Autodesk Fusion 360 part; units mm, degrees
sketch "Schizzo1" plane through (0, 0, 0) normal (0, 0, 1) x (1, 0, 0)
  line L0 (0, 0) -> (200, 0)
  line L1 (200, 0) -> (200, 200)
  line L2 (200, 200) -> (0, 200)
  line L3 (0, 200) -> (0, 0)
  line L4 (0, 100) -> (200, 100) construction
  line L5 (200, 100) -> (220, 100) construction
  line L6 (0, 100) -> (-20, 100) construction
  line L7 (220, 100) -> (220, 190.15)
  line L8 (220, 190.15) -> (200, 190.15)
  line L9 (220, 100) -> (220, 9.85)
  line L10 (220, 9.85) -> (200, 9.85)
  line L11 (-20, 100) -> (-20, 190.15)
  line L12 (-20, 190.15) -> (0, 190.15)
  line L13 (-20, 100) -> (-20, 9.85)
  line L14 (-20, 9.85) -> (0, 9.85)
  line L15 (0, 190.15) -> (200, 190.15) construction
  line L16 (200, 9.85) -> (0, 9.85) construction
  line L17 (0, 49.85) -> (200, 49.85) construction
  line L18 (122, 71.85) -> (78, 71.85)
  line L19 (78, 71.85) -> (78, 27.85)
  line L20 (78, 27.85) -> (122, 27.85)
  line L21 (122, 27.85) -> (122, 71.85)
  line L22 (122, 71.85) -> (78, 27.85) construction
  line L23 (78, 71.85) -> (122, 27.85) construction
  line L24 (23, 115) -> (17, 115)
  line L25 (17, 115) -> (17, 85)
  line L26 (17, 85) -> (23, 85)
  line L27 (23, 85) -> (23, 115)
  line L28 (23, 115) -> (17, 85) construction
  line L29 (17, 115) -> (23, 85) construction
  line L30 (183, 115) -> (177, 115)
  line L31 (177, 115) -> (177, 85)
  line L32 (177, 85) -> (183, 85)
  line L33 (183, 85) -> (183, 115)
  line L34 (183, 115) -> (177, 85) construction
  line L35 (177, 115) -> (183, 85) construction
  point P0 (100, 49.85)
  point P1 (20, 100)
  point P2 (180, 100)
  dimension "d1" = 200
  dimension "d2" = 200
  dimension "d3" = 180.3
  dimension "d4" = 20
  dimension "d10" = 40
  dimension "d11" = 44
  dimension "d12" = 44
  dimension "d15" = 20
  dimension "d16" = 20
  dimension "d17" = 30
  dimension "d18" = 6
  dimension "d19" = 6
  dimension "d20" = 30
extrude "Estrusione1" add sketch "Schizzo1" along normal blind 4
fillet "Raccordo1" radius 2 4 edges at (122, 27.85, 2) (78, 27.85, 2) (78, 71.85, 2) (122, 71.85, 2)
component "Component" placed x (1, 0, 0) y (0, 1, 0) z (0, 0, 1) at (0, 0, 0)
equation "d3 = 180 mm + 2 * t"
Can you work these out from the model? Positions are in its coordinate system, mm. Give positions to 0.01 mm unless a question says otherwise; leave off trailing zeros. Loops run counter-clockwise (first coordinate to the right, second up) from the corner with the lowest first, then second, coordinate; pieces in that order, holes last. Notation, with made-up numbers: M -32.5,-6 L -10.5,-6 A30 ccw -10.5,21 Z; hole C 59.5,-34.75 d2. An arc over 180 degrees is marked long. One line per question, with ' | ' between items. Start each with the question number.
Q1. If we section it at C-C (x = 116.5): Please give me the cut outline in (y, z), plus the area to 3 significant figures.
Q2. If we section it at D-D (x = -5): Please give me the cut outline in (y, z), plus the area to 3 significant figures.
Q3. If we section it at B-B (z = 1.2): Please give me the cut outline in (x, y).
Q4. For pin 1 Ø1.2 at (y, z) = (5.5, 3) entering from +X; pin 2 Ø1.2 at (x, z) = (-7, 3) entering from -Y, each with a flat end and sliding along its axis, tell me the tip position at first contact or that it passes through.
Q5. If we section it at A-A (y = 54): Please give me the cut outline in (x, z), plus the area to 3 significant figures.
Q6. If I drill on line 1 (Y direction, x = 91.5, z = 3.2); line 2 (X direction, y = 54.5, z = 3.25); line 3 (X direction, y = 105.5, z = 0.6), over which ranges is the centre line in solid material (lowest first)? Write a range as from..to.
Computed:
1) outline: M 0,0 L 27.85,0 L 27.85,4 L 0,4 Z; M 71.85,0 L 200,0 L 200,4 L 71.85,4 Z | area: 624 mm²
2) outline: M 9.85,0 L 190.15,0 L 190.15,4 L 9.85,4 Z | area: 721 mm²
3) outline: M -20,9.85 L 0,9.85 L 0,0 L 200,0 L 200,9.85 L 220,9.85 L 220,190.15 L 200,190.15 L 200,200 L 0,200 L 0,190.15 L -20,190.15 Z; hole M 17,85 L 23,85 L 23,115 L 17,115 Z; hole M 78,29.85 A2 ccw 80,27.85 L 120,27.85 A2 ccw 122,29.85 L 122,69.85 A2 ccw 120,71.85 L 80,71.85 A2 ccw 78,69.85 Z; hole M 177,85 L 183,85 L 183,115 L 177,115 Z
4) pin 1: stops at x = 200 | pin 2: stops at y = 9.85
5) outline: M -20,0 L 78,0 L 78,4 L -20,4 Z; M 122,0 L 220,0 L 220,4 L 122,4 Z | area: 784 mm²
6) line 1: y = 0..27.85, 71.85..200 | line 2: x = -20..78, 122..220 | line 3: x = -20..17, 23..177, 183..220
